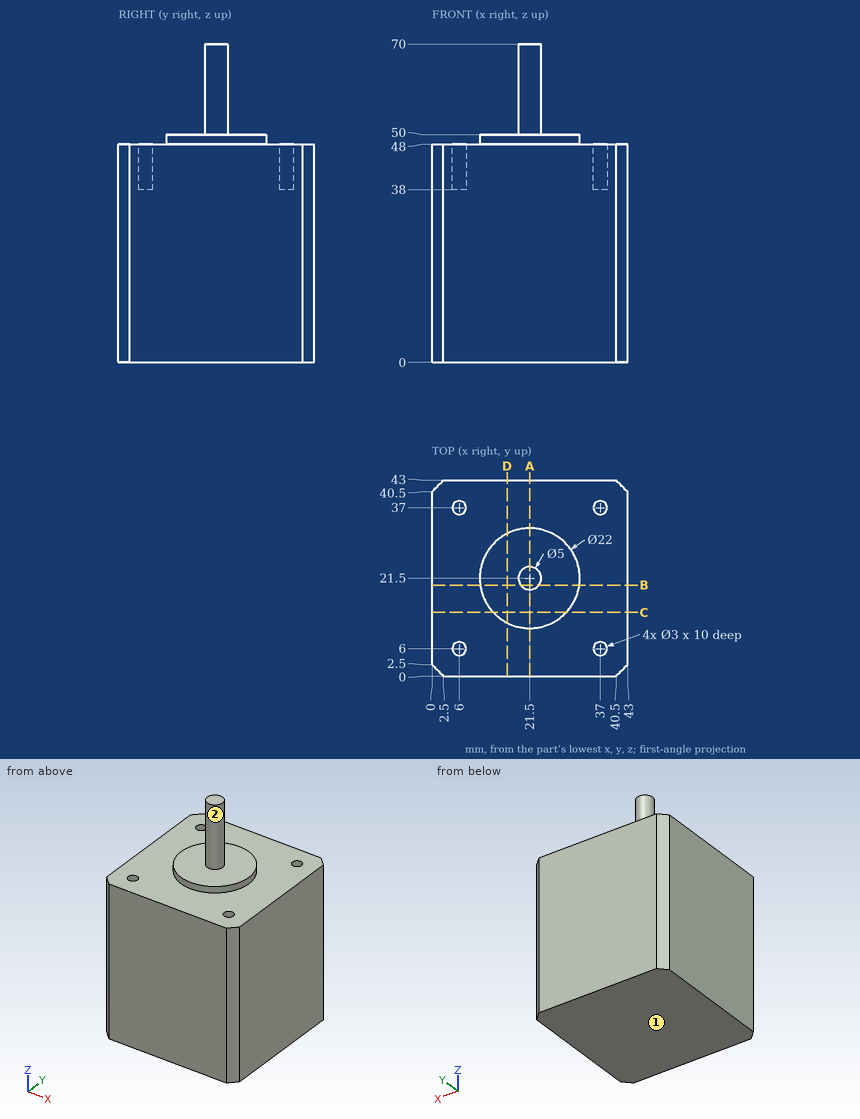
The drawing under review shows one solid part. Ordinate dimensions are in mm from its lowest x, y, z. A direction names the side the tool comes from. Coordinates: 2 decimals unless noted, no trailing zeros. Write each loop counter-clockwise with the first axis right and the second up, starting at its lowest first coordinate (ties: lowest second). Pieces come first, ordered by that corner, then holes. Notation, with made-up numbers: (84.25, 47.5) - (101.25, 47.5) arc R17 cw to (101.25, 70.5) - close; hole circle Ø6 at (64.25, 33). An arc over 180 degrees is marked (long way). Use one line per item in the form item = value.
Q1. Consider section D-D (x = 16.5). Write out the cut boundary in (y, z), plus the area to 3 significant figures.
Taken from the geometry:
outline = (0, 0) - (43, 0) - (43, 48) - (31.3, 48) - (31.3, 50) - (11.7, 50) - (11.7, 48) - (0, 48) - close
area = 2,100 mm^2
Q2. Consider section C-C (y = 14). Write out the cut boundary in (x, z).
Taken from the geometry:
outline = (0, 0) - (43, 0) - (43, 48) - (29.55, 48) - (29.55, 50) - (13.45, 50) - (13.45, 48) - (0, 48) - close
Q3. Insertion check: pin 1 Ø2.5 at (x, y) = (6.5, 5.5) entering from +Z; pin 2 Ø13 at (x, y) = (24.5, 31) entering from +Z; pin 3 Ø8 at (y, z) = (18, 52.5) entering from -X. Each pin has a flat end and moves straight along its axis. Give the tip position at first contact, or say it passes through.
Taken from the geometry:
pin_1 = 48
pin_2 = 50
pin_3 = 10.51
Q4. Consider section A-A (x = 21.5). Write out the cut boundary in (y, z).
Taken from the geometry:
outline = (0, 0) - (43, 0) - (43, 48) - (32.5, 48) - (32.5, 50) - (24, 50) - (24, 70) - (19, 70) - (19, 50) - (10.5, 50) - (10.5, 48) - (0, 48) - close
Q5. Consider section B-B (y = 20). Write out the cut boundary in (x, z), plus the area to 3 significant figures.
Taken from the geometry:
outline = (0, 0) - (43, 0) - (43, 48) - (32.4, 48) - (32.4, 50) - (23.5, 50) - (23.5, 70) - (19.5, 70) - (19.5, 50) - (10.6, 50) - (10.6, 48) - (0, 48) - close
area = 2,190 mm^2
Q6. For probe 1 along Y at (x, z) = (6, 42.25); probe 2 along Z at (x, y) = (28.5, 21.5); probe 3 along Z at (x, y) = (38.5, 32), list the stretches that pass through material, from the lowest coordinate up.
Taken from the geometry:
probe_1 = 0 to 4.5, 7.5 to 35.5, 38.5 to 43
probe_2 = 0 to 50
probe_3 = 0 to 48
Q7. Machinability: for the marked faces 1 and 2, which of the approach directions +Z, -Z, +X, -X, +Y, -Y give a long, thin tool a straight path to every point of the face, cutting with its end or side? Answer none if there is none.
Taken from the geometry:
face_1 = -Z, +X, -X, +Y, -Y
face_2 = +Z
